```python
from build123d import *

# Parameters (mm, degrees)
F1_DEPTH = 6.35
F0_R     = 1.5875
F2_DEPTH = 3.81


with BuildPart() as f1:
    # F0 (on Top) → F1 (new body)
    with BuildSketch(Plane.XY):
        with BuildLine():
            ThreePointArc((0.645552, 22.180257), (-1.275182, 22.425696), (-3.209795, 22.507705))
            ThreePointArc((-3.209795, 22.507705), (-5.144409, 22.425696), (-7.065142, 22.180257))
            ThreePointArc((-7.065142, 22.180257), (-12.645539, 20.469481), (-17.610809, 17.401308))
            Line((-17.610809, 17.401308), (-13.137701, 12.456375))
            ThreePointArc((-13.137701, 12.456375), (-8.4563, 14.980661), (-3.209795, 15.853424))
            ThreePointArc((-3.209795, 15.853424), (2.03671, 14.980661), (6.71811, 12.456375))
            Line((6.71811, 12.456375), (11.191218, 17.401308))
            ThreePointArc((11.191218, 17.401308), (6.225949, 20.469481), (0.645552, 22.180257))
        make_face()
        with BuildLine():
            Line((-14.247476, 11.51341), (-18.711746, 16.448572))
            ThreePointArc((-18.711746, 16.448572), (-24.501195, -8.674307), (-3.209795, -23.212295))
            ThreePointArc((-3.209795, -23.212295), (18.081605, -8.674307), (12.292155, 16.448572))
            Line((12.292155, 16.448572), (7.827885, 11.51341))
            ThreePointArc((7.827885, 11.51341), (12.805017, 2.127855), (10.899951, -8.323519))
            Line((10.899951, -8.323519), (2.17881, 0.229518))
            Line((2.17881, 0.229518), (-2.26534, 9.769376))
            Line((-2.26534, 9.769376), (-2.26534, -4.748298))
            Line((-2.26534, -4.748298), (6.48982, -13.334699))
            ThreePointArc((6.48982, -13.334699), (1.900789, -15.731088), (-3.209795, -16.558014))
            ThreePointArc((-3.209795, -16.558014), (-8.32038, -15.731088), (-12.90941, -13.334699))
            Line((-12.90941, -13.334699), (-4.154251, -4.748298))
            Line((-4.154251, -4.748298), (-4.154251, 9.769376))
            Line((-4.154251, 9.769376), (-8.5984, 0.229518))
            Line((-8.5984, 0.229518), (-17.319541, -8.323519))
            ThreePointArc((-17.319541, -8.323519), (-19.224607, 2.127855), (-14.247476, 11.51341))
        make_face()
    extrude(amount=F1_DEPTH)

    # F0 (on Top) → F2 (join)
    with BuildSketch(Plane.XY):
        with BuildLine():
            ThreePointArc((-7.065142, 22.180257), (-5.144409, 22.425696), (-3.209795, 22.507705))
            ThreePointArc((-3.209795, 22.507705), (-1.275182, 22.425696), (0.645552, 22.180257))
            ThreePointArc((0.645552, 22.180257), (-3.209795, 26.376933), (-7.065142, 22.180257))
        make_face()
        with Locations((-3.209795, 24.443971)):
            Circle(F0_R, mode=Mode.SUBTRACT)
        with BuildLine():
            ThreePointArc((12.292155, 16.448572), (11.749274, 16.933707), (11.191218, 17.401308))
            Line((11.191218, 17.401308), (6.71811, 12.456375))
            ThreePointArc((6.71811, 12.456375), (7.283595, 11.997365), (7.827885, 11.51341))
            Line((7.827885, 11.51341), (12.292155, 16.448572))
        make_face()
        with BuildLine():
            Line((-13.137701, 12.456375), (-17.610809, 17.401308))
            ThreePointArc((-17.610809, 17.401308), (-18.168864, 16.933707), (-18.711746, 16.448572))
            Line((-18.711746, 16.448572), (-14.247476, 11.51341))
            ThreePointArc((-14.247476, 11.51341), (-13.703186, 11.997365), (-13.137701, 12.456375))
        make_face()
    extrude(amount=F2_DEPTH)


solid = f1.part
```
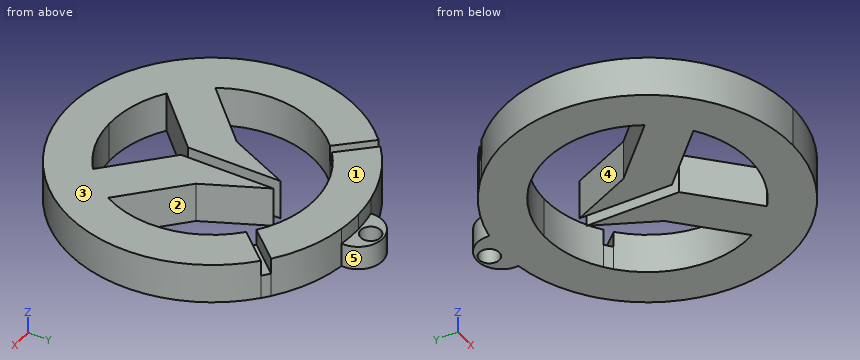
CAD build for the part. Positions are in the model's coordinates, mm. Face numbers are marked on the shaded views. A direction names the side the tool comes from. Round coordinates to 2 decimals unless told otherwise and drop trailing zeros. Write each loop counter-clockwise with the first axis right and the second up, starting at its lowest first coordinate (ties: lowest second). Pieces come first, ordered by that corner, then holes.
Item 1: Band-saw the part on B-B on z = 5.75. Write the cut outline in (x, y), then the cut area to 3 significant figures.
Filled in:
outline: (-18.71, 16.45) arc R22.86 ccw (long way) to (12.29, 16.45) - (7.83, 11.51) arc R16.21 cw to (10.9, -8.32) - (2.18, 0.23) - (-2.27, 9.77) - (-2.27, -4.75) - (6.49, -13.33) arc R16.21 cw to (-3.21, -16.56) arc R16.21 cw to (-12.91, -13.33) - (-4.15, -4.75) - (-4.15, 9.77) - (-8.6, 0.23) - (-17.32, -8.32) arc R16.21 cw to (-14.25, 11.51) - close; (-17.61, 17.4) - (-13.14, 12.46) arc R16.21 cw to (-3.21, 15.85) arc R16.21 cw to (6.72, 12.46) - (11.19, 17.4) arc R22.86 ccw to (0.65, 22.18) arc R22.86 ccw to (-3.21, 22.51) arc R22.86 ccw to (-7.07, 22.18) arc R22.86 ccw to start
area: 1,030 mm2
Item 2: Tool access for the marked faces 1 and 2: list every direction of +Z, -Z, +X, -X, +Y, -Y with a clear straight run to the whole face (end or side of a thin tool).
Filled in:
face 1: +Z, +X, -X, +Y, -Y
face 2: +Z, -Z
Item 3: Drop flat-ended pins along their axis: pin 1 Ø3.5 at (x, y) = (-4, 24.5) entering from +Z; pin 2 Ø10 at (x, y) = (-17, 3) entering from +Z; pin 3 Ø1 at (y, z) = (1, 2.5) entering from +X; pin 4 Ø1.9 at (y, z) = (4.5, 4) entering from +X. Give the stop position or say it passes through.
Filled in:
pin 1: stops at z = 3.81
pin 2: stops at z = 6.35
pin 3: stops at x = 19.63
pin 4: stops at x = 19.31
Item 4: Band-saw the part on D-D on z = 1. Write the cut outline in (x, y) (1 decimal).
Filled in:
outline: (-18.7, 16.4) arc R22.9 ccw (long way) to (12.3, 16.4) arc R22.9 ccw to (11.2, 17.4) arc R22.9 ccw to (0.6, 22.2) arc R3.9 ccw (long way) to (-7.1, 22.2) arc R22.9 ccw to (-17.6, 17.4) arc R22.9 ccw to start; hole (-17.3, -8.3) - (-8.6, 0.2) - (-4.2, 9.8) - (-4.2, -4.7) - (-12.9, -13.3) arc R16.2 ccw to (-3.2, -16.6) arc R16.2 ccw to (6.5, -13.3) - (-2.3, -4.7) - (-2.3, 9.8) - (2.2, 0.2) - (10.9, -8.3) arc R16.2 ccw to (7.8, 11.5) arc R16.2 ccw to (6.7, 12.5) arc R16.2 ccw to (-3.2, 15.9) arc R16.2 ccw to (-13.1, 12.5) arc R16.2 ccw to (-14.2, 11.5) arc R16.2 ccw to start; hole circle Ø3.2 at (-3.2, 24.4)
Item 5: Band-saw the part on C-C on x = -10. Write the cut outline in (y, z).
Filled in:
outline: (-22.18, 0) - (-15.07, 0) - (-15.07, 6.35) - (-22.18, 6.35) - close; (-10.48, 0) - (-1.15, 0) - (-1.15, 6.35) - (-10.48, 6.35) - close; (14.36, 0) - (21.48, 0) - (21.48, 6.35) - (14.36, 6.35) - close
Item 6: Band-saw the part on A-A on y = 1. Write the cut outline in (x, z), then the cut area to 3 significant figures.
Filled in:
outline: (-26.03, 0) - (-19.36, 0) - (-19.36, 6.35) - (-26.03, 6.35) - close; (-8.24, 0) - (-4.15, 0) - (-4.15, 6.35) - (-8.24, 6.35) - close; (-2.27, 0) - (1.82, 0) - (1.82, 6.35) - (-2.27, 6.35) - close; (12.94, 0) - (19.61, 0) - (19.61, 6.35) - (12.94, 6.35) - close
area: 137 mm2
Item 7: Mould opens along X. For the marked faces 3, 4 and 5 say: released by +X, released by -X, zero draft, split by the parting line, or undercut.
Filled in:
face 3: zero draft
face 4: undercut
face 5: split by the parting line
Item 8: Drill centre lines: L1, parallel to Y at x = -3, z = 1.25; L2, parallel to Y at x = -15, z = 5; L3, parallel to X at y = 1, z = 4. Where is each one in solid material? Low to high.
Filled in:
L1: y = -23.21 to -16.56, 15.85 to 22.87, 26.02 to 26.37
L2: y = -19.94 to -6.05, 10.77 to 12.35, 14.52 to 19.23
L3: x = -26.03 to -19.36, -8.24 to -4.15, -2.27 to 1.82, 12.94 to 19.61
